Could you check a few things on this model? Use its own coordinates, in mm. A direction names the side the tool comes from. Give positions to 0.01 mm unless a question says otherwise; leave off trailing zeros. Write each loop counter-clockwise with the first axis right and the second up, starting at its lowest first coordinate (ties: lowest second). Pieces come first, ordered by that corner, then holes. Notation, with made-up numbers: (-22, -37.5) - (29, -37.5) arc R19 ccw to (29, -5.5) - close; hole circle Ø8 at (-24, -36). An arc over 180 degrees is marked (long way). Write item = value, one per line.
Autodesk Inventor part; units mm, degrees
ref_plane "YZ Plane" through (0, 0, 0) normal (1, 0, 0) x (0, 1, 0)
ref_plane "XZ Plane" through (0, 0, 0) normal (0, 1, 0) x (-1, 0, 0)
ref_plane "XY Plane" through (0, 0, 0) normal (0, 0, 1) x (1, 0, 0)
sketch "Sketch1" plane through (0, 0, 0) normal (0, 0, 1) x (1, 0, 0)
  line L0 (-11.999, -0.0009) -> (209.001, -0.0009) construction
  circle A0 centre (47.001, -0.0009) radius 42.5 construction
  circle A1 centre (132.001, -0.0009) radius 42.5 construction
  circle A2 centre (47.001, -0.0009) radius 47.5625 construction
  circle A3 centre (132.001, -0.0009) radius 47.5625 construction
  arc A4 (82.1177, 32.0773) -> (-0.5615, -0.0019) centre (47.001, -0.0009) ccw
  arc A5 (179.5635, -0.0009) -> (96.8843, 32.0773) centre (132.001, -0.0009) ccw
  arc A6 (-0.5615, -0.0019) -> (82.1177, -32.079) centre (47.001, -0.0009) ccw
  arc A7 (96.8843, -32.079) -> (179.5635, -0.0009) centre (132.001, -0.0009) ccw
  arc A8 (75.7238, 47.5616) -> (-8.5615, -0.0015) centre (47.001, -0.0009) ccw
  arc A9 (187.5635, -0.0009) -> (103.2782, 47.5616) centre (132.001, -0.0009) ccw
  line L1 (47.001, 47.5616) -> (132.001, 47.5616) construction
  arc A10 (75.7238, 47.5616) -> (103.2782, 47.5616) centre (89.501, 70.3754) ccw
  arc A11 (-8.5615, -0.0015) -> (75.7238, -47.5634) centre (47.001, -0.0009) ccw
  arc A12 (103.2782, -47.5634) -> (75.7238, -47.5634) centre (89.501, -70.3772) ccw
  arc A13 (103.2782, -47.5634) -> (187.5635, -0.0009) centre (132.001, -0.0009) ccw
  arc A14 (82.1177, 32.0773) -> (96.8843, 32.0773) centre (89.501, 38.8217) ccw
  line L2 (82.1177, 32.0773) -> (96.8843, 32.0773) construction
  arc A15 (96.8843, -32.079) -> (82.1177, -32.079) centre (89.501, -38.8234) ccw
  point P0 (0, 0)
  point P1 (89.501, 21.3519)
  point P2 (46.9513, 55.5616)
  point P3 (132.0501, 55.5616)
  dimension "d0" = 221
  dimension "d1" = 85
  dimension "d2" = 85
  dimension "d3" = 85
  dimension "d4" = 95.125
  dimension "d5" = 95.125
  dimension "d6" = 8
  dimension "d7" = 10
extrude "Extrusion1" add sketch "Sketch1" along normal blind 1.5
equation "\"d2\" = d1"
equation "\"d3\" = d1"
equation "\"d5\" = d4"
properties part number "Dichtung" material "Rubber, Silicone"
1. Thinking about a two-plate mould opening in X: for faces 1 (the face through (148.457, 44.624, 0.74)), 2 (the face through (89, 29, 0)), which applies, pulls with the +X half, pulls with the -X half, needs draft (parallel to the pull), parting line crosses it, or undercut?
Filled sheet:
face_1 = undercut
face_2 = needs draft
2. If we section it at C-C, the plane z = 1.05: Please give me the cut outline in (x, y) (1 decimal), and give its area (3 significant figures).
Filled sheet:
outline = (-8.6, 0) arc R55.6 ccw to (75.7, -47.6) arc R26.7 cw to (103.3, -47.6) arc R55.6 ccw to (187.6, 0) arc R55.6 ccw to (103.3, 47.6) arc R26.7 cw to (75.7, 47.6) arc R55.6 ccw to start; hole (-0.6, 0) arc R47.6 ccw to (82.1, -32.1) arc R10 cw to (96.9, -32.1) arc R47.6 ccw to (179.6, 0) arc R47.6 ccw to (96.9, 32.1) arc R10 cw to (82.1, 32.1) arc R47.6 ccw to start
area = 4,260 mm2
3. If we section it at B-B, the plane y = 14.5: Please give me the cut outline in (x, z).
Filled sheet:
outline = (-6.64, 0) - (1.7, 0) - (1.7, 1.5) - (-6.64, 1.5) - close; (177.3, 0) - (185.64, 0) - (185.64, 1.5) - (177.3, 1.5) - close
4. If we section it at D-D, the plane y = 41.5: Please give me the cut outline in (x, z).
Filled sheet:
outline = (10.06, 0) - (23.77, 0) - (23.77, 1.5) - (10.06, 1.5) - close; (70.24, 0) - (108.77, 0) - (108.77, 1.5) - (70.24, 1.5) - close; (155.24, 0) - (168.95, 0) - (168.95, 1.5) - (155.24, 1.5) - close
5. If we section it at A-A, the plane x = 20: Please give me the cut outline in (y, z), and give its area (3 significant figures).
Filled sheet:
outline = (-48.56, 0) - (-39.16, 0) - (-39.16, 1.5) - (-48.56, 1.5) - close; (39.15, 0) - (48.56, 0) - (48.56, 1.5) - (39.15, 1.5) - close
area = 28.2 mm2
6. For pin 1 (8 mm diameter, centred on x = 153.5, y = -38.5, fed in from -Z), with a flat end and sliding along its axis, tell me the tip position at first contact or that it passes through.
Filled sheet:
pin_1 = 0
7. I need wall thicknesses on line 1 (Y direction, x = 131, z = 1); line 2 (X direction, y = 40.5, z = 1.25); line 3 (X direction, y = 41, z = 1.1). Which ranges of each line are inside material? Lowest first, please.
Filled sheet:
line_1 = -55.55 to -47.55, 47.55 to 55.55
line_2 = 8.96 to 22.06, 71.94 to 107.06, 156.94 to 170.04
line_3 = 9.5 to 22.89, 71.11 to 107.89, 156.11 to 169.5
8. Which directions (+Z, -Z, +X, -X, +Y, -Y) give clear straight access to the entire face, cutting with the end or side of a thin tool? Please do faces 3 (the face through (89.704, 43.725, 0.74)), 4 (the face through (29.054, 44.046, 0.74)).
Filled sheet:
face_3 = +Z, -Z, +Y
face_4 = +Z, -Z
